from build123d import *

# Parameters (mm, degrees)
ESQUISSE1_R             = 152
ESQUISSE1_R_2           = 150
BOSS_EXTRU_1_DEPTH      = 700
ESQUISSE2_R             = 152
BOSS_EXTRU_2_DEPTH      = 1
ESQUISSE6_W             = 304
ESQUISSE6_H             = 150
ENL_V_MAT_EXTRU_3_DEPTH = 152
ESQUISSE7_R             = 1.5
ENL_V_MAT_EXTRU_4_DEPTH = 240
ESQUISSE8_R             = 3
ESQUISSE8_R_2           = 1
ESQUISSE8_W             = 28
ESQUISSE8_H             = 20
ENL_V_MAT_EXTRU_5_DEPTH = 220
ESQUISSE9_R             = 1
ENL_V_MAT_EXTRU_6_DEPTH = 170
ESQUISSE10_R            = 1
ENL_V_MAT_EXTRU_8_DEPTH = 220


with BuildPart() as part:
    # Esquisse1 → Boss.-Extru.1 (new body)
    with BuildSketch(Plane(origin=(0, 0, 0), x_dir=(1, 0, 0), z_dir=(0, 1, 0))):
        with Locations(Location((0, 0, 0), (0, 0, 270))):
            Circle(ESQUISSE1_R)
        with Locations(Location((0, 0, 0), (0, 0, 270))):
            Circle(ESQUISSE1_R_2, mode=Mode.SUBTRACT)
    extrude(amount=-BOSS_EXTRU_1_DEPTH)

    # Esquisse2 → Boss.-Extru.2 (add)
    with BuildSketch(Plane(origin=(0, -700, 0), x_dir=(-1, 0, 0), z_dir=(0, -1, 0))):
        with Locations(Location((0, 0, 0), (0, 0, 270))):
            Circle(ESQUISSE2_R)
    extrude(amount=BOSS_EXTRU_2_DEPTH)

    # Esquisse6 → Enlèv. mat.-Extru.3 (cut)
    with BuildSketch(Plane.XY):
        with Locations((0, -625)):
            Rectangle(ESQUISSE6_W, ESQUISSE6_H)
    extrude(amount=ENL_V_MAT_EXTRU_3_DEPTH, mode=Mode.SUBTRACT)

    # Esquisse7 → Enlèv. mat.-Extru.4 (cut)
    with BuildSketch(Plane(origin=(0, 0, 0), x_dir=(0, 0, -1), z_dir=(1, 0, 0))):
        with Locations(Location((-15, -44, 0), (0, 0, 180))):
            Circle(ESQUISSE7_R)
        with Locations(Location((15, -44, 0), (0, 0, 180))):
            Circle(ESQUISSE7_R)
        with BuildLine():
            Line((-4, 0), (-14, 0))
            Line((-14, 0), (-14, -36))
            Line((-14, -36), (14, -36))
            Line((14, -36), (14, 0))
            Line((14, 0), (4, 0))
            ThreePointArc((4, 0), (0, -4), (-4, 0))
        make_face()
    extrude(amount=ENL_V_MAT_EXTRU_4_DEPTH, mode=Mode.SUBTRACT)


with BuildPart() as enl_v_mat_extru_4_kept_piece:
    # of the separate pieces the step leaves, the one the design keeps (enl_v_mat_extru_4_pieces_kept)
    add(part.part.solids().sort_by_distance((0, 0, 152))[0])

    # Esquisse8 → Enlèv. mat.-Extru.5 (cut)
    with BuildSketch(Plane(origin=(0, 0, 0), x_dir=(0, 0, -1), z_dir=(1, 0, 0))):
        with Locations(Location((0, -200, 0), (0, 0, 180))):
            Circle(ESQUISSE8_R)
        with Locations(Location((-14, -162, 0), (0, 0, 180))):
            Circle(ESQUISSE8_R_2)
        with Locations(Location((14, -162, 0), (0, 0, 180))):
            Circle(ESQUISSE8_R_2)
        with Locations((0, -178)):
            Rectangle(ESQUISSE8_W, ESQUISSE8_H)
    extrude(amount=ENL_V_MAT_EXTRU_5_DEPTH, mode=Mode.SUBTRACT)

    # Esquisse9 → Enlèv. mat.-Extru.6 (cut)
    with BuildSketch(Plane(origin=(0, 0, 0), x_dir=(0, 0, -1), z_dir=(1, 0, 0))):
        with Locations((0, -200)):
            Circle(ESQUISSE9_R)
    extrude(amount=-ENL_V_MAT_EXTRU_6_DEPTH, mode=Mode.SUBTRACT)

    # Esquisse10 → Enlèv. mat.-Extru.8 (cut)
    with BuildSketch(Plane(origin=(0, 0, 0), x_dir=(0, 0, -1), z_dir=(1, 0, 0))):
        with Locations((-45, -70)):
            Circle(ESQUISSE10_R)
        with Locations((45, -70)):
            Circle(ESQUISSE10_R)
    extrude(amount=-ENL_V_MAT_EXTRU_8_DEPTH, mode=Mode.SUBTRACT)


solid = enl_v_mat_extru_4_kept_piece.part
Can you work these out from the model? Positions are in its coordinate system, mm. A direction names the side the tool comes from. Coordinates: 2 decimals unless noted, no trailing zeros. Loops run counter-clockwise (first coordinate to the right, second up) from the corner with the lowest first, then second, coordinate; pieces in that order, holes last. Notation, with made-up numbers: (59, -21.75) - (99, -21.75) arc R19 cw to (99, 5.25) - close; hole circle Ø11 at (88, -18.5). An arc over 180 degrees is marked (long way). Put each result on its own line as item: value. Start each with the question number.
Item 1: Which directions (+Z, -Z, +X, -X, +Y, -Y) give clear straight access to the entire face, cutting with the end or side of a thin tool? Please do faces 4 (the face through (-23, -550, 149)), 5 (the face through (-2, -701, -2)).
Item 2: If I drill on line 1 along Y through (x, z) = (-144.05, -45); line 2 along X through (y, z) = (-525, 29.5); line 3 along X through (y, z) = (-186.5, 117.5), over which ranges is the centre line in solid material (lowest first)?
Item 3: Suppose I cut it at C-C (y = -337). Please give me the cut outline in (x, z).
Item 4: If we mould it in two halves opening along Z, with no side actions, what happens to faces 1 (the face through (6.595, -345.1, -149.855)), 2 (the face through (-2, -700, -1)), 3 (the face through (-6.683, -345.593, -151.853))? For each: +Z half, -Z half, draft (parallel to the pull), parting line (faces both ways), or undercut.
Item 5: Suppose I cut it at D-D (z = -66). Please give me the cut outline in (x, y).
Item 6: Suppose I cut it at A-A (x = 0). Please give me the cut outline in (y, z).
Item 7: For pin 1 (6 mm diameter, centred on y = -206, z = 9, fed in from +X); pin 2 (2.5 mm diameter, centred on y = -70, z = 45, fed in from +X); pin 3 (2 mm diameter, centred on x = -151.5, y = -645, fed in from +Z), each with a flat end and sliding along its axis, tell me the tip position at first contact or that it passes through.
Item 8: Suppose I cut it at B-B (z = 32). Please give me the cut outline in (x, y), and give its area (3 significant figures).
Here are the results:
1. face 4: +Z, +X, -X
1. face 5: +Z, -Z, +X, -X, -Y
2. line 1: -701 to -71, -69 to 0
2. line 2: -149.11 to -147.07, 147.07 to 149.11
2. line 3: -96.42 to -93.24, 93.24 to 96.42
3. outline: circle Ø304 at (0, 0); hole circle Ø300 at (0, 0)
4. face 1: undercut
4. face 2: draft
4. face 3: parting line
5. outline: (-136.92, -701) - (136.92, -701) - (136.92, 0) - (134.7, 0) - (134.7, -700) - (-134.7, -700) - (-134.7, 0) - (-136.92, 0) - close
6. outline: (-701, -152) - (0, -152) - (0, -150) - (-700, -150) - (-700, 152) - (-701, 152) - close; (-550, 150) - (0, 150) - (0, 152) - (-550, 152) - close
7. pin 1: x = 151.88
7. pin 2: x = 145.57
7. pin 3: z = 0
8. outline: (-148.59, -701) - (148.59, -701) - (148.59, -700) - (-148.59, -700) - close; (-148.59, -550) - (-146.55, -550) - (-146.55, 0) - (-148.59, 0) - close; (146.55, -550) - (148.59, -550) - (148.59, 0) - (146.55, 0) - close
8. area: 2,550 mm²
